from build123d import *

# Parameters (mm, degrees)
SKETCH1_R           = 3.175
BOSS_EXTRUDE1_DEPTH = 96.52
SKETCH2_R           = 5.08
BOSS_EXTRUDE2_DEPTH = 2.54
BOSS_EXTRUDE3_DEPTH = 193.04


with BuildPart() as part:
    # Sketch1 → Boss-Extrude1 (new body)
    with BuildSketch(Plane.XY):
        Circle(SKETCH1_R)
    boss_extrude1 = extrude(amount=BOSS_EXTRUDE1_DEPTH)

    # Sketch2 → Boss-Extrude2 (add)
    with BuildSketch(Plane.XY.offset(96.52)):
        Circle(SKETCH2_R)
    boss_extrude2 = extrude(amount=-BOSS_EXTRUDE2_DEPTH)

    # Mirror1: Boss-Extrude1, Boss-Extrude2 across plane
    add(boss_extrude1.mirror(Plane.XY))
    add(boss_extrude2.mirror(Plane.XY))

    # Sketch3 → Boss-Extrude3 (add, through all)
    with BuildSketch(Plane(origin=(0, 0, -96.52), x_dir=(-1, 0, 0), z_dir=(0, 0, -1))):
        with BuildLine():
            Line((-1.27, 4.91868885), (-1.27, 2.199704526))
            Line((-1.27, 2.199704526), (1.27, 2.199704526))
            Line((1.27, 2.199704526), (1.27, 4.91868885))
            Line((1.27, 4.91868885), (1.27, 6.221703947))
            ThreePointArc((1.27, 6.221703947), (0, 6.35), (-1.27, 6.221703947))
            Line((-1.27, 6.221703947), (-1.27, 4.91868885))
        make_face()
        with BuildLine():
            Line((1.69959174, 1.887587857), (2.484494906, -0.528095695))
            Line((2.484494906, -0.528095695), (5.070402665, 0.312116669))
            Line((5.070402665, 0.312116669), (6.309643664, 0.714770478))
            ThreePointArc((6.309643664, 0.714770478), (6.039208878, 1.962257914), (5.524740498, 3.130454029))
            Line((5.524740498, 3.130454029), (4.285499499, 2.72780022))
            Line((4.285499499, 2.72780022), (1.69959174, 1.887587857))
        make_face()
        with BuildLine():
            Line((2.320405462, -1.033111073), (0.265502297, -2.526085614))
            Line((0.265502297, -2.526085614), (1.863681184, -4.72579014))
            Line((1.863681184, -4.72579014), (2.629574241, -5.779951497))
            ThreePointArc((2.629574241, -5.779951497), (3.732436352, -5.137257914), (4.684477407, -4.286976956))
            Line((4.684477407, -4.286976956), (3.918584349, -3.232815599))
            Line((3.918584349, -3.232815599), (2.320405462, -1.033111073))
        make_face()
        with BuildLine():
            Line((-0.265502297, -2.526085614), (-2.320405462, -1.033111073))
            Line((-2.320405462, -1.033111073), (-3.918584349, -3.232815599))
            Line((-3.918584349, -3.232815599), (-4.684477407, -4.286976956))
            ThreePointArc((-4.684477407, -4.286976956), (-3.732436352, -5.137257914), (-2.629574241, -5.779951497))
            Line((-2.629574241, -5.779951497), (-1.863681184, -4.72579014))
            Line((-1.863681184, -4.72579014), (-0.265502297, -2.526085614))
        make_face()
        with BuildLine():
            Line((-2.484494906, -0.528095695), (-1.69959174, 1.887587857))
            Line((-1.69959174, 1.887587857), (-4.285499499, 2.72780022))
            Line((-4.285499499, 2.72780022), (-5.524740498, 3.130454029))
            ThreePointArc((-5.524740498, 3.130454029), (-6.039208878, 1.962257914), (-6.309643664, 0.714770478))
            Line((-6.309643664, 0.714770478), (-5.070402665, 0.312116669))
            Line((-5.070402665, 0.312116669), (-2.484494906, -0.528095695))
        make_face()
    extrude(amount=-BOSS_EXTRUDE3_DEPTH)


solid = part.part
Source: CAD feature listing. Evaluate the final solid. Frame: model axes, mm. Round coordinates to 2 decimals unless told otherwise and drop trailing zeros. One line per item, written item: value. Start each with the question number.
Item 1: Ray query, L1, parallel to Z at x = 0.5, y = -4.75; L2, parallel to X at y = 1, z = -29.5; L3, parallel to X at y = 3.75, z = 8. Return the intervals inside material, ascending. Write a range as from..to.
Item 2: Mould query, pull axis Z, two halves, no side actions, for faces 1 (the flat face through (1.27, 5, -1)), 2 (the flat face through (0, 0, 96.52)), 3 (the flat face through (0, 0, -96.52)). Classes: pulls with the +Z half, pulls with the -Z half, needs draft (parallel to the pull), parting line crosses it, or undercut.
Item 3: Pin query (flat end, axial travel): pin 1 (1.5 mm diameter, centred on y = 4.5, z = 64, fed in from -X); pin 2 (1 mm diameter, centred on y = 5, z = 56.5, fed in from +X); pin 3 (1.5 mm diameter, centred on x = -4, z = -50, fed in from -Y). Return the tip coordinate at first contact, or that it passes through.
Result set:
1. L1: z = -96.52..-93.98, 93.98..96.52
1. L2: x = -6.27..6.27
1. L3: x = -1.27..1.27
2. face 1: undercut
2. face 2: pulls with the +Z half
2. face 3: pulls with the -Z half
3. pin 1: stops at x = -1.27
3. pin 2: stops at x = 1.27
3. pin 3: stops at y = -5.46
